Autodesk Inventor part; units mm, degrees
ref_plane "YZ Plane" through (0, 0, 0) normal (1, 0, 0) x (0, 1, 0)
ref_plane "XZ Plane" through (0, 0, 0) normal (0, 1, 0) x (-1, 0, 0)
ref_plane "XY Plane" through (0, 0, 0) normal (0, 0, 1) x (1, 0, 0)
sketch "Sketch1" plane through (0, 0, 0) normal (0, 0, 1) x (1, 0, 0)
  line L0 (0, 0) -> (-25.7, 0)
  line L1 (-25.7, 0) -> (-25.7, -35)
  line L2 (-25.7, -35) -> (0, -35)
  line L3 (0, -35) -> (0, 0)
  line L4 (-25.7, 0) -> (-23.52, 0)
  line L5 (-23.52, 0) -> (-23.52, -7.65)
  line L6 (-23.52, -7.65) -> (-25.7, -7.65)
  line L7 (-25.7, -7.65) -> (-25.7, 0)
  line L8 (-8.88, 0) -> (-17.72, 0)
  line L9 (-17.72, 0) -> (-17.72, -1.6)
  line L10 (-17.72, -1.6) -> (-8.88, -1.6)
  line L11 (-8.88, -1.6) -> (-8.88, 0)
  circle A0 centre (-24.2, -27.7) radius 0.5
  circle A1 centre (-24.2, -25.2) radius 0.5
  circle A2 centre (-24.2, -22.7) radius 0.5
  circle A3 centre (-24.2, -20.2) radius 0.5
  circle A4 centre (-24.2, -17.7) radius 0.5
  circle A5 centre (-24.2, -15.2) radius 0.5
  circle A6 centre (-24.2, -12.7) radius 0.5
  circle A7 centre (-24.2, -10.2) radius 0.5
  line L12 (-12.85, -35) -> (-12.85, 0) construction
  circle A8 centre (-1.5, -27.7) radius 0.5
  circle A9 centre (-1.5, -25.2) radius 0.5
  circle A10 centre (-1.5, -22.7) radius 0.5
  circle A11 centre (-1.5, -20.2) radius 0.5
  circle A12 centre (-1.5, -17.7) radius 0.5
  circle A13 centre (-1.5, -15.2) radius 0.5
  circle A14 centre (-1.5, -12.7) radius 0.5
  circle A15 centre (-1.5, -10.2) radius 0.5
  line L13 (-23.4, -35) -> (-25.7, -32.7)
  line L14 (-2.3, -35) -> (0, -32.7)
  dimension "d0" = 25.7
  dimension "d1" = 35
  dimension "d4" = 2.18
  dimension "d5" = 7.65
  dimension "d7" = 5.8
  dimension "d8" = 8.88
  dimension "d9" = 1.6
  dimension "d10" = 1
  dimension "d11" = 1.5
  dimension "d12" = 7.3
  dimension "d15" = 2.5
  dimension "d20" = 2.3
  dimension "d21" = 2.3
extrude "Extrusion2" add sketch "Sketch1" along normal blind 1.13 contours L3 L14 L2 L13 L1 L6 L5 L0 L9 L10 L11
ref_plane "Work Plane1" through (-17.72, -0.7, 0) normal (0, 1, 0) x (1, 0, 0)
sketch "Sketch2" plane through (-17.72, -0.7, 0) normal (0, 1, 0) x (1, 0, 0)
  line L0 (8.84, 0) -> (0, 0)
  line L1 (0, 0) -> (0, -1.13)
  line L2 (8.84, -1.13) -> (0, -1.13)
  line L3 (8.84, 0) -> (8.84, -1.13)
  line L4 (8.205, -4.13) -> (0.635, -4.13)
  line L5 (0.635, -4.13) -> (0.635, -1.13)
  line L6 (0.635, -1.13) -> (8.205, -1.13)
  line L7 (8.205, -1.13) -> (8.205, -4.13)
  point P0 (17.72, 0)
  point P1 (4.42, -4.13)
  point P2 (4.42, -1.13)
  dimension "d25" = 7.57
  dimension "d26" = 3
  dimension "d27" = 0
  dimension "d28" = 0
extrude "Extrusion3" add sketch "Sketch2" against normal blind 5.5 contours L7 L4 L5 L2
sketch "Sketch3" plane through (0, 0, 0) normal (0, 0, -1) x (-1, 0, 0)
  line L0 (21.1, -10.55) -> (5.1, -10.55)
  line L1 (5.1, -10.55) -> (5.1, -35.5)
  line L2 (5.1, -35.5) -> (21.1, -35.5)
  line L3 (21.1, -35.5) -> (21.1, -10.55)
  line L4 (0, 0) -> (8.88, 0)
  line L5 (0, -32.7) -> (0, 0)
  line L6 (23.4, -35) -> (2.3, -35)
  point P0 (5.1, -35)
  point P1 (21.1, -35)
  dimension "d31" = 10.55
  dimension "d32" = 16
  dimension "d33" = 5.1
  dimension "d34" = 0.5
extrude "Extrusion4" add sketch "Sketch3" along normal blind 1
sketch "Sketch4" plane through (0, 0, -1) normal (0, 0, -1) x (-1, 0, 0)
  line L0 (19.1, -12.6) -> (7.1, -12.6)
  line L1 (7.1, -12.6) -> (7.1, -27.7)
  line L2 (7.1, -27.7) -> (19.1, -27.7)
  line L3 (19.1, -27.7) -> (19.1, -12.6)
  line L4 (5.1, -35.5) -> (21.1, -35.5)
  line L5 (21.1, -35.5) -> (21.1, -10.55)
  point P0 (0, 0)
  dimension "d37" = 12
  dimension "d38" = 15.1
  dimension "d39" = 7.8
  dimension "d40" = 2
extrude "Extrusion5" add sketch "Sketch4" along normal blind 2.3
sketch "Sketch5" plane through (0, 0, 1.13) normal (0, 0, 1) x (1, 0, 0)
  line L0 (-23.52, 0) -> (-23.52, -7.65)
  line L1 (-23.52, -1.7) -> (-21.27, -1.7)
  line L2 (-21.27, -1.7) -> (-21.27, -6.2)
  line L3 (-21.27, -6.2) -> (-23.52, -6.2)
  line L4 (-23.52, -6.2) -> (-23.52, -1.7)
  line L5 (-17.72, 0) -> (-23.52, 0)
  line L6 (-20.5, -16.49) -> (-16.9, -16.49)
  line L7 (-16.9, -16.49) -> (-16.9, -28.69)
  line L8 (-16.9, -28.69) -> (-20.5, -28.69)
  line L9 (-20.5, -28.69) -> (-20.5, -16.49)
  line L10 (-23.4, -35) -> (-2.3, -35)
  line L11 (-25.7, -7.65) -> (-25.7, -32.7)
  line L12 (-19.06, -9.55) -> (-8.96, -9.55)
  line L13 (-8.96, -9.55) -> (-8.96, -16.84)
  line L14 (-8.96, -16.84) -> (-19.06, -16.84)
  line L15 (-19.06, -16.84) -> (-19.06, -9.55)
  line L16 (-5.1, -35.5) -> (-21.1, -35.5)
  line L17 (-14.4, -17.28) -> (-10.7, -17.28)
  line L18 (-10.7, -17.28) -> (-10.7, -28.94)
  line L19 (-10.7, -28.94) -> (-14.4, -28.94)
  line L20 (-14.4, -28.94) -> (-14.4, -17.28)
  line L21 (-8.2009, -5.539) -> (-2.3, -5.539)
  line L22 (-2.3, -5.539) -> (-2.3, -10.0071)
  line L23 (-2.3, -10.0071) -> (-8.2009, -10.0071)
  line L24 (-8.2009, -10.0071) -> (-8.2009, -5.539)
  point P0 (0, 0)
  point P1 (-22.395, -1.7)
  point P2 (-16.9, -16.84)
  point P3 (-19.06, -16.49)
  dimension "d43" = 1.7
  dimension "d44" = 2.25
  dimension "d45" = 4.5
  dimension "d46" = 6.31
  dimension "d47" = 3.6
  dimension "d48" = 5.2
  dimension "d49" = 12.2
  dimension "d50" = 6.64
  dimension "d51" = 7.29
  dimension "d52" = 18.66
  dimension "d53" = 6.56
  dimension "d54" = 11.66
  dimension "d55" = 3.7
  dimension "d56" = 15
  dimension "d57" = 10.1
extrude "Extrusion6" add sketch "Sketch5" along normal blind 1.85 contours L1 L2 L3 L0
extrude "Extrusion7" add sketch "Sketch5" along normal blind 1.1 contours L6 L15 L14 L7 L8 L9 | L17 L18 L19 L20 | L21 L22 L23 L24
extrude "Extrusion8" add sketch "Sketch5" along normal blind 1.6 contours L15 L12 L13 L14 L7 L6 | L6 L7 L14 L15
sketch "Sketch6" plane through (0, 0, -1) normal (0, 0, -1) x (-1, 0, 0)
  line L0 (8.6, -28.04) -> (5.6, -28.04)
  line L1 (5.6, -28.04) -> (5.6, -29.74)
  line L2 (5.6, -29.74) -> (8.6, -29.74)
  line L3 (8.6, -29.74) -> (8.6, -28.04)
  line L4 (5.1, -35.5) -> (21.1, -35.5)
  line L5 (5.1, -10.55) -> (5.1, -35.5)
  point P0 (0, 0)
  dimension "d64" = 3
  dimension "d65" = 5.76
  dimension "d66" = 1.7
  dimension "d67" = 0.5
extrude "Extrusion9" add sketch "Sketch6" along normal blind 0.65
properties part number "ESP-12F"
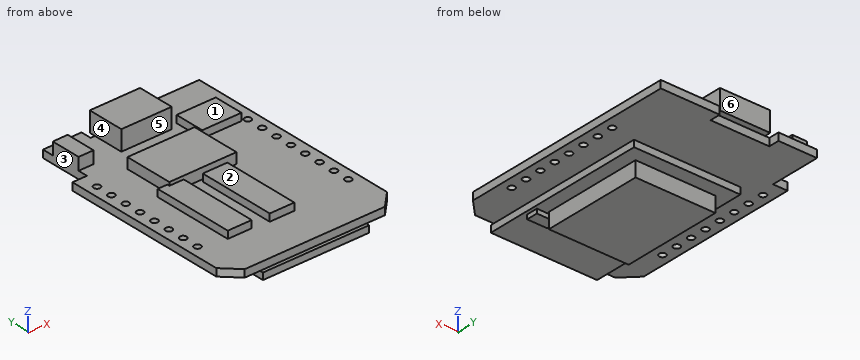
Build history of the part. All positions in model axes, mm. Face numbers are marked on the shaded views. A direction names the side the tool comes from. Round coordinates to 2 decimals unless told otherwise and drop trailing zeros. Loops run counter-clockwise (first coordinate to the right, second up) from the corner with the lowest first, then second, coordinate; pieces in that order, holes last. Notation, with made-up numbers: (-19, -22.75) -> (0, -22.75) arc R17 cw to (0, -11.75) -> close; hole circle Ø6 at (63, 66.25). An arc over 180 degrees is marked (long way). Use CSV: the item, a comma, the result in double quotes. Start each with the question number.
Q1. Which spindle directions (+Z, -Z, +X, -X, +Y, -Y) get a long thin tool onto all of the face, cutting with end or side? Do the marked faces 1, 2 and 3. Say none if no direction does.
Q2. Drill centre lines: L1, parallel to Y at x = -14.5, z = 1.25; L2, parallel to X at y = -27.5, z = 1.25; L3, parallel to Z at x = -8, y = -12.5. Where is each one in solid material? Low to high.
Q3. Flat gauge pins, fed straight in: pin 1 Ø0.6 at (x, z) = (-5.5, 2) entering from +Y; pin 2 Ø1.5 at (y, z) = (-4, 2.5) entering from +X (3 decimals); pin 3 Ø0.6 at (y, z) = (-0.5, 0.5) entering from -X. Where does each tip first touch, or does it go through?
Q4. Mould opens along Y. For the marked faces 4, 5 and 6 say: +Y half, -Y half, draft (parallel to the pull), parting line (faces both ways), or undercut.
Q5. Saw through at C-C on y = -26.5. Give the cut face in (x, z), and give its area (3 significant figures).
Q6. Saw through at A-A on y = -15.2. Give the cut face in (x, z), and give its area (3 significant figures).
Q7. Saw through at B-B on z = 0.5. Count the separate pieces of the cut face and the enclosed holes in it, and give its area (3 significant figures).
Solutions:
1,face 1,"+Z, +X, +Y, -Y"
1,face 2,"+Z, +X, -X, -Y"
1,face 3,"+Z, -Z, -X, +Y"
2,L1,"y = -16.84 to -9.55, -6.2 to -0.7"
2,L2,"x = -20.5 to -16.9, -14.4 to -10.7"
2,L3,"z = -1 to 1.13"
3,pin 1,"stops at y = -5.54"
3,pin 2,"stops at x = -9.515"
3,pin 3,"stops at x = -23.52"
4,face 4,"draft"
4,face 5,"undercut"
4,face 6,"+Y half"
5,outline,"(-25.7, 0) -> (-21.1, 0) -> (-21.1, -1) -> (-19.1, -1) -> (-19.1, -3.3) -> (-7.1, -3.3) -> (-7.1, -1) -> (-5.1, -1) -> (-5.1, 0) -> (0, 0) -> (0, 1.13) -> (-10.7, 1.13) -> (-10.7, 2.23) -> (-14.4, 2.23) -> (-14.4, 1.13) -> (-16.9, 1.13) -> (-16.9, 2.23) -> (-20.5, 2.23) -> (-20.5, 1.13) -> (-25.7, 1.13) -> close"
5,area,"80.7 mm^2"
6,outline,"(-25.7, 0) -> (-24.7, 0) -> (-24.7, 1.13) -> (-25.7, 1.13) -> close; (-23.7, 0) -> (-21.1, 0) -> (-21.1, -1) -> (-19.1, -1) -> (-19.1, -3.3) -> (-7.1, -3.3) -> (-7.1, -1) -> (-5.1, -1) -> (-5.1, 0) -> (-2, 0) -> (-2, 1.13) -> (-8.96, 1.13) -> (-8.96, 2.73) -> (-19.06, 2.73) -> (-19.06, 1.13) -> (-23.7, 1.13) -> close; (-1, 0) -> (0, 0) -> (0, 1.13) -> (-1, 1.13) -> close"
6,area,"86.5 mm^2"
7,separate pieces,"1"
7,enclosed holes,"16"
7,area,"851 mm^2"
